Could you check a few things on this drawing? It's one solid part, dimensions in mm from its lowest x, y, z. A direction names the side the tool comes from. Round coordinates to 2 decimals unless told otherwise and drop trailing zeros. Order: outer loops, then holes, each group sorted by start corner. A loop starts at its lowest first (then second) coordinate and runs counter-clockwise, first axis right, second up. Notation, with made-up numbers: M 10.25,44.25 L 55.25,44.25 A14 cw 55.25,70.25 Z; hole C 47.5,-38 d4. An arc over 180 degrees is marked long. Answer as a JSON object with one key per item and string values. Group by question number.
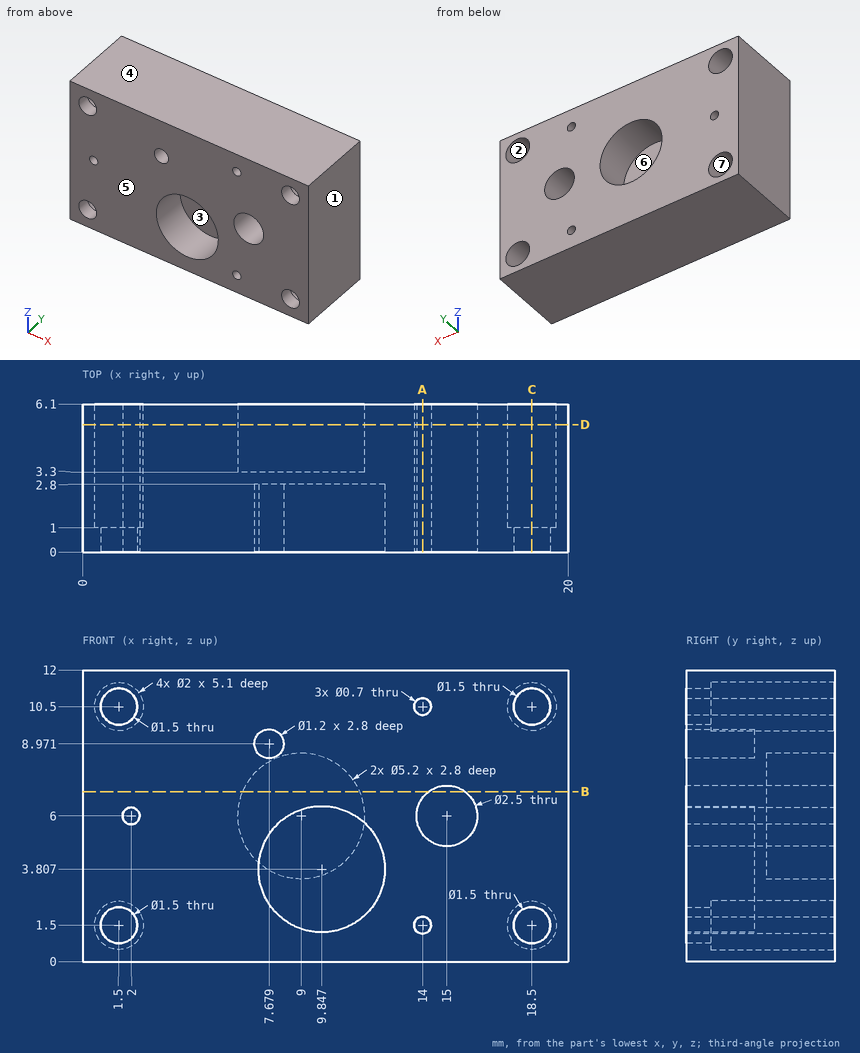
1) If we section it at D-D on y = 5.25: Count the separate pieces of the cut face and the enclosed holes in it, plus the area to 3 significant figures.
2) If we section it at B-B on z = 7: Write out the boundary of the cut face in (x, y).
3) For pin 1 (4 mm diameter, centred on x = 9, z = 6, fed in from +Y); pin 2 (4 mm diameter, centred on x = 10, z = 4, fed in from -Y); pin 3 (1.6 mm diameter, centred on x = 18.5, z = 1.5, fed in from +Y), each with a flat end and sliding along its axis, tell me the tip position at first contact or that it passes through.
4) If we section it at C-C on x = 18.5: Write out the boundary of the cut face in (y, z), plus the area to 3 significant figures.
5) I need wall thicknesses on line 1 along X through (y, z) = (4.3, 1.5); line 2 along X through (y, z) = (4.75, 6); line 3 along Z through (x, y) = (2.25, 2.25) (1 decimal). Which ranges of each line are inside material? Lowest first, please.
6) If we section it at A-A on x = 14: Write out the boundary of the cut face in (y, z).
7) We'd pull the mould along Z, two halves only. Please class the marked faces 4, 5, 6 and 7: +Z half, -Z half, draft (parallel to the pull), parting line (faces both ways), or undercut.
8) Which directions (+Z, -Z, +X, -X, +Y, -Y) give clear straight access to the entire face, cutting with the end or side of a thin tool? Please do the marked faces 1, 2 and 3.
Findings:
{
 "1": {"separate pieces": "1", "enclosed holes": "9", "area": "200 mm^2"},
 "2": {"outline": "M 0,0 L 14.25,0 L 14.25,6.1 L 11.4,6.1 L 11.4,3.3 L 6.6,3.3 L 6.6,6.1 L 0,6.1 Z; M 15.75,0 L 20,0 L 20,6.1 L 15.75,6.1 Z"},
 "3": {"pin 1": "stops at y = 3.3", "pin 2": "stops at y = 2.8", "pin 3": "stops at y = 1"},
 "4": {"outline": "M 0,0 L 6.1,0 L 6.1,0.5 L 1,0.5 L 1,0.75 L 0,0.75 Z; M 0,2.25 L 1,2.25 L 1,2.5 L 6.1,2.5 L 6.1,9.5 L 1,9.5 L 1,9.75 L 0,9.75 Z; M 0,11.25 L 1,11.25 L 1,11.5 L 6.1,11.5 L 6.1,12 L 0,12 Z", "area": "49.8 mm^2"},
 "5": {"line 1": "x = 0 to 0.5, 2.5 to 13.65, 14.35 to 17.5, 19.5 to 20", "line 2": "x = 0 to 1.65, 2.35 to 6.4, 11.6 to 13.75, 16.25 to 20", "line 3": "z = 0 to 0.8, 2.2 to 5.8, 6.2 to 9.8, 11.2 to 12"},
 "6": {"outline": "M 0,0 L 6.1,0 L 6.1,1.15 L 0,1.15 Z; M 0,1.85 L 6.1,1.85 L 6.1,5.25 L 0,5.25 Z; M 0,6.75 L 6.1,6.75 L 6.1,10.15 L 0,10.15 Z; M 0,10.85 L 6.1,10.85 L 6.1,12 L 0,12 Z"},
 "7": {"face 4": "+Z half", "face 5": "draft", "face 6": "undercut", "face 7": "undercut"},
 "8": {"face 1": "+Z, -Z, +X, +Y, -Y", "face 2": "+Y", "face 3": "-Y"}
}
